Input: part model. Units: mm. Frame: model coordinates. A direction names the side the tool comes from. Round coordinates to 2 decimals unless told otherwise and drop trailing zeros. Loops run counter-clockwise (first coordinate to the right, second up) from the corner with the lowest first, then second, coordinate; pieces in that order, holes last. Notation, with made-up numbers: M -26.75,-16.5 L -13.75,-16.5 A31 cw -13.75,19.5 Z; hole C 79.5,20 d8. An arc over 180 degrees is marked long. Put each result on its own line as item: value. Start each with the question number.
1) Pin query (flat end, axial travel): pin 1 (6 mm diameter, centred on y = 192.5, z = 20, fed in from +X); pin 2 (4.5 mm diameter, centred on x = -7.5, y = 100, fed in from -Z); pin 3 (2 mm diameter, centred on y = 100, z = 160, fed in from +X); pin 4 (1.5 mm diameter, centred on y = 100, z = 110, fed in from +X). Return the tip coordinate at first contact, or that it passes through.
2) Reachability of faces 4 (the face through (0, 101, 144)), 5 (the face through (-3.5, 107.2, 80.4)) from +Z, -Z, +X, -X, +Y, -Y: full face, straight path, thin tool, end or side. Return the list, or none.
3) Draft query along Y for faces 1 (the face through (-15, 101, 144)), 2 (the face through (-7.975, 27.187, 269.754)), 3 (the face through (-7, 200, 144)). Return one class per face: +Y half, -Y half, draft (parallel to the pull), parting line (faces both ways), or undercut.
4) Line query: probe 1 along Y at (x, z) = (-4, 142.5); probe 2 along Z at (x, y) = (-9.25, 192.5); probe 3 along Y at (x, z) = (-3, 185). Output: solid intervals per line, ascending.
5) Section A-A on z = 142.5. Output: boundary loops of the cut face in (x, y), plus the area to 4 significant figures.
from build123d import *

# Parameters (mm, degrees)
SKETCH1_W                    = 285
SKETCH1_H                    = 200
BOSS_EXTRUDE1_DEPTH          = 15
SKETCH4_R                    = 3
CUT_EXTRUDE1_DEPTH           = 7
M6_TAPPED_HOLE1_D            = 5
M6_TAPPED_HOLE1_DEPTH        = 10
M6_TAPPED_HOLE1_TIP          = 1.502151548
LPATTERN1_COUNT              = 6
LPATTERN1_PITCH              = 25
M6_TAPPED_HOLE2_D            = 5
M6_TAPPED_HOLE2_DEPTH        = 10
M6_TAPPED_HOLE2_TIP          = 1.502151548
M4_TAPPED_HOLE1_D            = 3.3
M4_TAPPED_HOLE1_DEPTH        = 10.1
M4_TAPPED_HOLE1_TIP          = 0.991420021
M10_TAPPED_HOLE1_D           = 8.5
M10_TAPPED_HOLE1_CSINK_D     = 10
M10_TAPPED_HOLE1_CSINK_ANGLE = 90
F_6_5_6_5_DIAMETER_HOLE1_D   = 6.5


with BuildPart() as part:
    # Sketch1 → Boss-Extrude1 (new body)
    with BuildSketch(Plane(origin=(0, 0, 0), x_dir=(0, 0, -1), z_dir=(1, 0, 0))):
        with Locations((-142.5, 100)):
            Rectangle(SKETCH1_W, SKETCH1_H)
    extrude(amount=-BOSS_EXTRUDE1_DEPTH)

    # Sketch4 → Cut-Extrude1 (cut)
    with BuildSketch(Plane(origin=(0, 0, 0), x_dir=(0, 0, -1), z_dir=(1, 0, 0))):
        with Locations((-217, 109)):
            Circle(SKETCH4_R)
        with Locations((-78, 109)):
            Circle(SKETCH4_R)
    extrude(amount=-CUT_EXTRUDE1_DEPTH, mode=Mode.SUBTRACT)

    # M6 Tapped Hole1
    with Locations(Plane(origin=(0, 0, 0), x_dir=(-1, 0, 0), z_dir=(0, 0, -1))):
        with Locations((7.5, 25), (7.5, 100), (7.5, 175)):
            Hole(M6_TAPPED_HOLE1_D / 2, depth=M6_TAPPED_HOLE1_DEPTH)
            with Locations((0, 0, -(M6_TAPPED_HOLE1_DEPTH + M6_TAPPED_HOLE1_TIP / 2))):  # 118° drill point
                Cone(0, M6_TAPPED_HOLE1_D / 2, M6_TAPPED_HOLE1_TIP, mode=Mode.SUBTRACT)

    # Sketch5 → M3 Tapped Hole1 (revolve, cut)
    with BuildSketch(Plane(origin=(0, 100, 85), x_dir=(0, 0, -1), z_dir=(0, 1, 0))):
        Polygon((0, 0), (0, 8.251075774), (1.25, 7.5), (1.25, 0), align=None)
    m3_tapped_hole1 = revolve(axis=Axis((6.35, 100, 85), (-1, 0, 0)), mode=Mode.SUBTRACT)

    # LPattern1: M3 Tapped Hole1 ×6
    with Locations(*[(0, 0, i * LPATTERN1_PITCH) for i in range(1, LPATTERN1_COUNT)]):
        add(m3_tapped_hole1, mode=Mode.SUBTRACT)

    # M6 Tapped Hole2
    with Locations(Plane(origin=(0, 0, 0), x_dir=(0, 0, -1), z_dir=(1, 0, 0))):
        with Locations((-47, 58), (-47, 142)):
            Hole(M6_TAPPED_HOLE2_D / 2, depth=M6_TAPPED_HOLE2_DEPTH)
            with Locations((0, 0, -(M6_TAPPED_HOLE2_DEPTH + M6_TAPPED_HOLE2_TIP / 2))):  # 118° drill point
                Cone(0, M6_TAPPED_HOLE2_D / 2, M6_TAPPED_HOLE2_TIP, mode=Mode.SUBTRACT)

    # M4 Tapped Hole1
    with Locations(Plane(origin=(0, 0, 0), x_dir=(0, 0, -1), z_dir=(1, 0, 0))):
        with Locations((-276, 81), (-276, 99)):
            Hole(M4_TAPPED_HOLE1_D / 2, depth=M4_TAPPED_HOLE1_DEPTH)
            with Locations((0, 0, -(M4_TAPPED_HOLE1_DEPTH + M4_TAPPED_HOLE1_TIP / 2))):  # 118° drill point
                Cone(0, M4_TAPPED_HOLE1_D / 2, M4_TAPPED_HOLE1_TIP, mode=Mode.SUBTRACT)

    # M10 Tapped Hole1 (through all)
    with Locations(Plane(origin=(0, 0, 0), x_dir=(0, 0, -1), z_dir=(1, 0, 0))):
        with Locations((-274, 27), (-274, 173)):
            CounterSinkHole(M10_TAPPED_HOLE1_D / 2, M10_TAPPED_HOLE1_CSINK_D / 2, counter_sink_angle=M10_TAPPED_HOLE1_CSINK_ANGLE)

    # Ø6.5 (6.5) Diameter Hole1 (through all)
    with Locations(Plane(origin=(0, 0, 0), x_dir=(0, 0, -1), z_dir=(1, 0, 0))):
        with Locations((-265, 7.5), (-142.5, 7.5), (-20, 7.5), (-20, 192.5), (-142.5, 192.5), (-265, 192.5)):
            Hole(F_6_5_6_5_DIAMETER_HOLE1_D / 2)


solid = part.part
Geometry results:
1. pin 1: passes through
1. pin 2: stops at z = 10.15
1. pin 3: stops at x = -7.65
1. pin 4: stops at x = -7.8
2. face 4: +Z, -Z, +X, +Y, -Y
2. face 5: +X
3. face 1: draft
3. face 2: undercut
3. face 3: +Y half
4. probe 1: y = 0 to 4.25, 10.75 to 189.25, 195.75 to 200
4. probe 2: z = 0 to 16.75, 23.25 to 139.25, 145.75 to 261.75, 268.25 to 285
4. probe 3: y = 0 to 98.75, 101.25 to 200
5. outline: M -15,0 L 0,0 L 0,4.25 L -15,4.25 Z; M -15,10.75 L 0,10.75 L 0,189.25 L -15,189.25 Z; M -15,195.75 L 0,195.75 L 0,200 L -15,200 Z
5. area: 2,805 mm²
